The drawing under review shows one solid part. Ordinate dimensions are in mm from its lowest x, y, z. Coordinates: 2 decimals unless noted, no trailing zeros. Write each loop counter-clockwise with the first axis right and the second up, starting at its lowest first coordinate (ties: lowest second). Pieces come first, ordered by that corner, then holes.
Q1. To check wall thickness, follow probe 1 along Y at (x, z) = (3, 57.95); probe 2 along Y at (x, z) = (2.9, 51.5); probe 3 along Y at (x, z) = (1.7, 16.5). State the ranges of each line that lie inside material, in increasing order.
Q2. Add section A-A, the plane y = 3. Give the boundary of the cut face in (x, z), plus the area to 3 significant figures.
Q3. Clearance check with flat-ended pins moving along their axes: pin 1 Ø1 at (y, z) = (2, 27.5) entering from +X; pin 2 Ø1 at (x, z) = (1, 34) entering from +Y; pin 3 Ø2 at (y, z) = (4.5, 40.5) entering from -X. State where each tip first meets the part, or that it passes through.
Q4. Add section D-D, the plane y = 5.4. Give the boundary of the cut face in (x, z).
Q5. Add section C-C, the plane z = 34.5. Give the boundary of the cut face in (x, y).
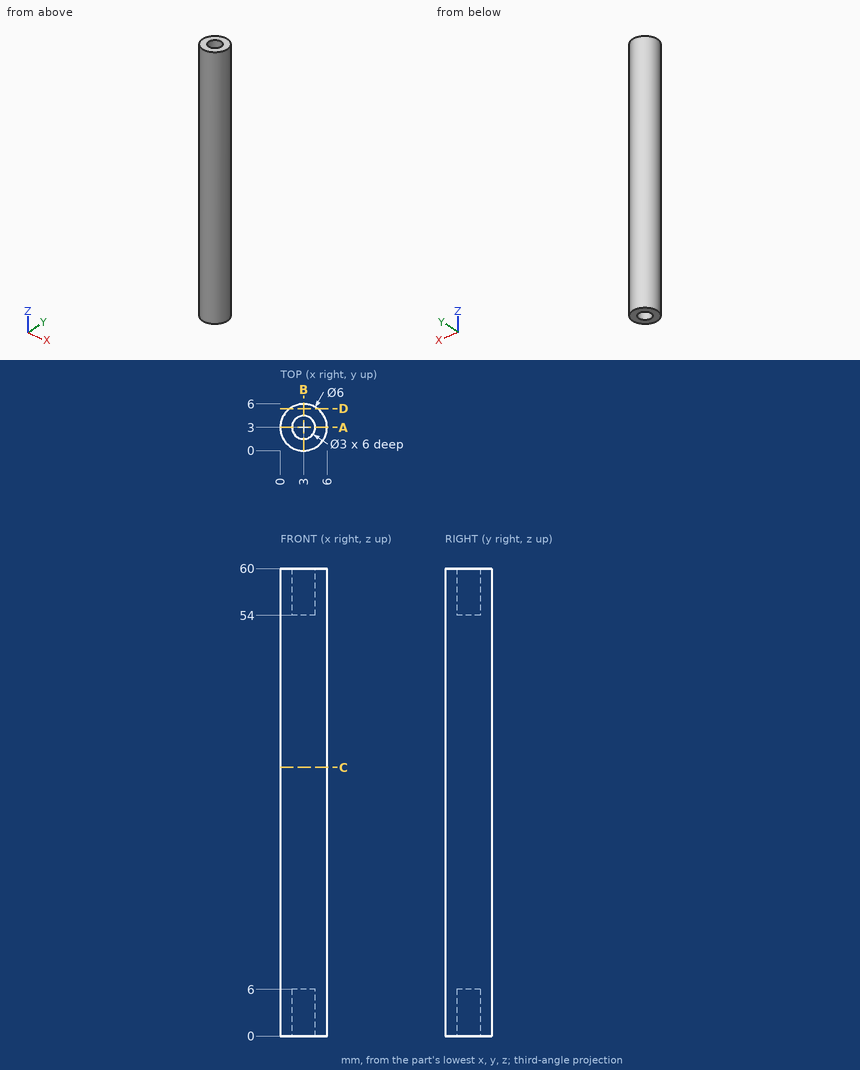
Here are the results:
1. probe 1: y = 0 to 1.5, 4.5 to 6
1. probe 2: y = 0 to 6
1. probe 3: y = 0.3 to 5.7
2. outline: (0, 0) - (1.5, 0) - (1.5, 6) - (4.5, 6) - (4.5, 0) - (6, 0) - (6, 60) - (4.5, 60) - (4.5, 54) - (1.5, 54) - (1.5, 60) - (0, 60) - close
2. area: 324 mm2
3. pin 1: stops at x = 5.96
3. pin 2: stops at y = 5.6
3. pin 3: stops at x = 0.04
4. outline: (1.2, 0) - (4.8, 0) - (4.8, 60) - (1.2, 60) - close
5. outline: circle Ø6 at (3, 3)
